```python
from build123d import *

# Parameters (mm, degrees)
SKETCH1_R           = 4.7625
BOSS_EXTRUDE1_DEPTH = 3.175


with BuildPart() as part:
    # Sketch1 → Boss-Extrude1 (new body)
    with BuildSketch(Plane.XY):
        with BuildLine():
            Line((111.332808166, 350.586079181), (63.710529936, 415.237184501))
            ThreePointArc((63.710529936, 415.237184501), (62.634536999, 416.513021087), (61.400531956, 417.636743182))
            Line((61.400531956, 417.636743182), (17.210961523, 385.086518286))
            ThreePointArc((17.210961523, 385.086518286), (14.359037805, 381.713915243), (13.335, 377.417490362))
            Line((13.335, 377.417490362), (13.335, 267.002909993))
            ThreePointArc((13.335, 267.002909993), (18.563575119, 258.501947797), (28.509038477, 259.333882069))
            Line((28.509038477, 259.333882069), (95.90843461, 308.980562961))
            Line((95.90843461, 308.980562961), (112.073002649, 336.647282747))
            ThreePointArc((112.073002649, 336.647282747), (113.789568713, 343.727489431), (111.332808166, 350.586079181))
        make_face()
        with Locations((35.56, 302.837639338)):
            Circle(SKETCH1_R, mode=Mode.SUBTRACT)
        with Locations((35.56, 347.287639338)):
            Circle(SKETCH1_R, mode=Mode.SUBTRACT)
    extrude(amount=BOSS_EXTRUDE1_DEPTH)


solid = part.part
```
Work out the finished part from the listing and answer in its coordinate system (mm). Round coordinates to 2 decimals unless told otherwise and drop trailing zeros. Order: outer loops, then holes, each group sorted by start corner. A loop starts at its lowest first (then second) coordinate and runs counter-clockwise, first axis right, second up.
Q1. Given pin 1 Ø1 at (x, z) = (84.5, 1) entering from +Y; pin 2 Ø1.5 at (x, z) = (102, 1.5) entering from +Y, each flat-ended and moving along its own axis, determine where each tip first touches the part or whether it passes through.
Solution:
pin 1: stops at y = 387.69
pin 2: stops at y = 364.27
Q2. Find the intervals of material crossed by line 1 along Y through (x, z) = (35.56, 2.2); line 2 along Y through (x, z) = (34.5, 2.45); line 3 along Y through (x, z) = (107.5, 2.45), in increasing order.
Solution:
line 1: y = 264.53 to 298.08, 307.6 to 342.53, 352.05 to 398.6
line 2: y = 263.75 to 298.19, 307.48 to 342.64, 351.93 to 397.82
line 3: y = 328.82 to 355.79
Q3. A cutting plane is placed at C-C, the plane y = 295. Determine the outline of the cut face in (x, z) (3 decimals).
Solution:
outline: (13.335, 0) - (76.929, 0) - (76.929, 3.175) - (13.335, 3.175) - close
Q4. A cutting plane is placed at A-A, the plane x = 35.56. Determine the outline of the cut face in (y, z) (1 decimal).
Solution:
outline: (264.5, 0) - (298.1, 0) - (298.1, 3.2) - (264.5, 3.2) - close; (307.6, 0) - (342.5, 0) - (342.5, 3.2) - (307.6, 3.2) - close; (352.1, 0) - (398.6, 0) - (398.6, 3.2) - (352.1, 3.2) - close
Q5. A cutting plane is placed at D-D, the plane x = 74. Determine the outline of the cut face in (y, z) (3 decimals), then the cut area to 3 significant figures.
Solution:
outline: (292.843, 0) - (401.268, 0) - (401.268, 3.175) - (292.843, 3.175) - close
area: 344 mm2
Q6. A cutting plane is placed at B-B, the plane z = 1.2. Count the separate pieces of the cut face and the enclosed holes in it, then the cut area to 3 significant figures.
Solution:
separate pieces: 1
enclosed holes: 2
area: 10,200 mm2
Q7. The mould has two halves that part along X. Classify faces 1 (the flat face through (13.335, 323, 2)), 2 (the cylindrical face through (40.1, 348.72, 1.57)), 3 (the flat face through (61.74, 283.81, 1.57)), 4 (the cylindrical face through (18.43, 258.57, 1.57)): pulls with the +X half, pulls with the -X half, needs draft (parallel to the pull), parting line crosses it, or undercut.
Solution:
face 1: pulls with the -X half
face 2: undercut
face 3: pulls with the +X half
face 4: parting line crosses it
